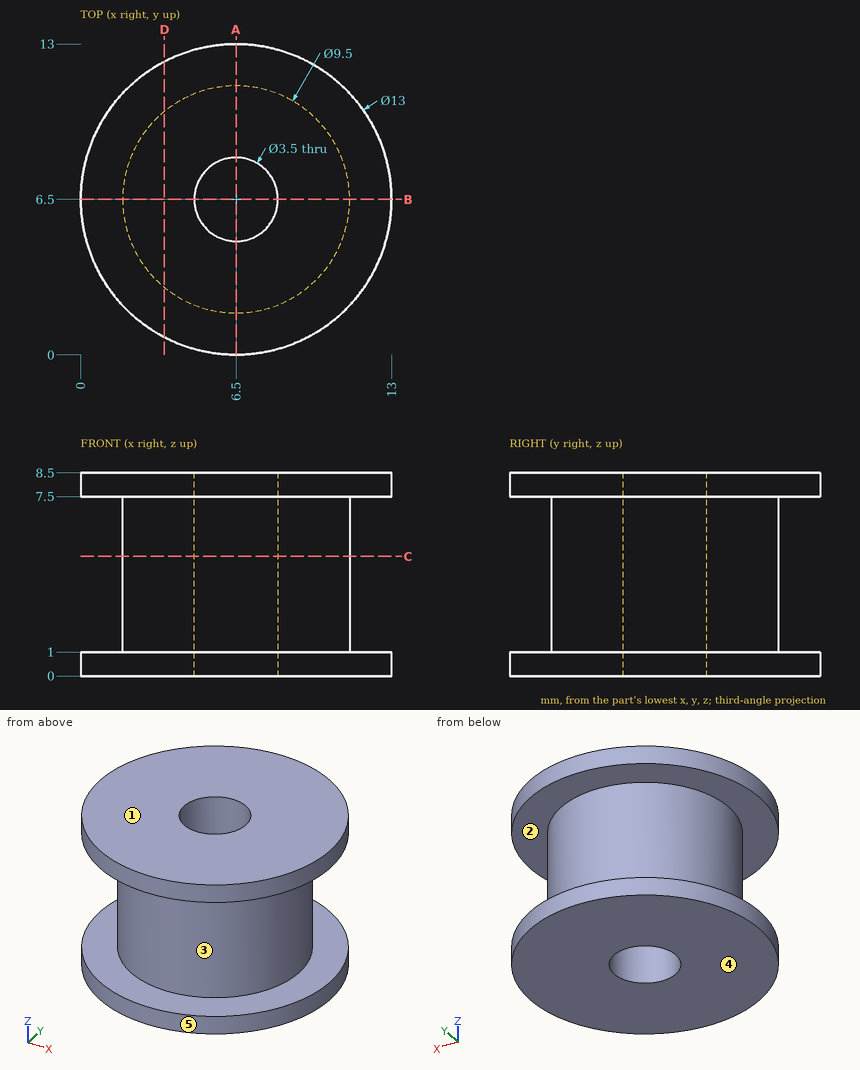
Study the drawing (mm; zero at the part's minimum x, y, z) and answer. A direction names the side the tool comes from. Coordinates: 2 decimals unless noted, no trailing zeros. Write each loop counter-clockwise with the first axis right and the second up, starting at its lowest first coordinate (ties: lowest second). Pieces come first, ordered by that corner, then holes.
Q1. Section C-C, the plane z = 5 is taken. Write down the section's boundary in (x, y), then the cut area to 3 significant figures.
Returned:
outline: circle Ø9.5 at (6.5, 6.5); hole circle Ø3.5 at (6.5, 6.5)
area: 61.3 mm2
Q2. Find the intervals of material crossed by line 1 along Z through (x, y) = (12.5, 7.5); line 2 along Y through (x, z) = (6.5, 6.5); line 3 along Y through (x, z) = (8, 2.5), in increasing order.
Returned:
line 1: z = 0 to 1, 7.5 to 8.5
line 2: y = 1.75 to 4.75, 8.25 to 11.25
line 3: y = 1.99 to 5.6, 7.4 to 11.01
Q3. Which of the six approach directions +Z, -Z, +X, -X, +Y, -Y give full straight-line access (tool end or side, diameter ignored) to the marked faces 1 and 2?
Returned:
face 1: +Z, +X, -X, +Y, -Y
face 2: none
Q4. Section D-D, the plane x = 3.5 is taken. Write down the section's boundary in (y, z).
Returned:
outline: (0.73, 0) - (12.27, 0) - (12.27, 1) - (10.18, 1) - (10.18, 7.5) - (12.27, 7.5) - (12.27, 8.5) - (0.73, 8.5) - (0.73, 7.5) - (2.82, 7.5) - (2.82, 1) - (0.73, 1) - close
Q5. Section A-A, the plane x = 6.5 is taken. Write down the section's boundary in (y, z), then the cut area to 3 significant figures.
Returned:
outline: (0, 0) - (4.75, 0) - (4.75, 8.5) - (0, 8.5) - (0, 7.5) - (1.75, 7.5) - (1.75, 1) - (0, 1) - close; (8.25, 0) - (13, 0) - (13, 1) - (11.25, 1) - (11.25, 7.5) - (13, 7.5) - (13, 8.5) - (8.25, 8.5) - close
area: 58.0 mm2
Q6. Given P1, Ø2, axis at x = 8, z = 4, coming from the +Y side; P2, Ø5, axis at x = 11, y = 11, coming from the -Z side; P3, Ø1.5, axis at x = 10, z = 2.5, coming from the -Y side; P4, Ø4, axis at y = 3.5, z = 3.5, coming from the -X side, each flat-ended and moving along its own axis, determine where each tip first touches the part or whether it passes through.
Returned:
P1: stops at y = 11.22
P2: stops at z = 0
P3: stops at y = 2.63
P4: stops at x = 1.86
Q7. The mould has two halves that part along Z. Classify the marked faces 3, 4 and 5: released by +Z, released by -Z, zero draft, split by the parting line, or undercut.
Returned:
face 3: undercut
face 4: released by -Z
face 5: zero draft
